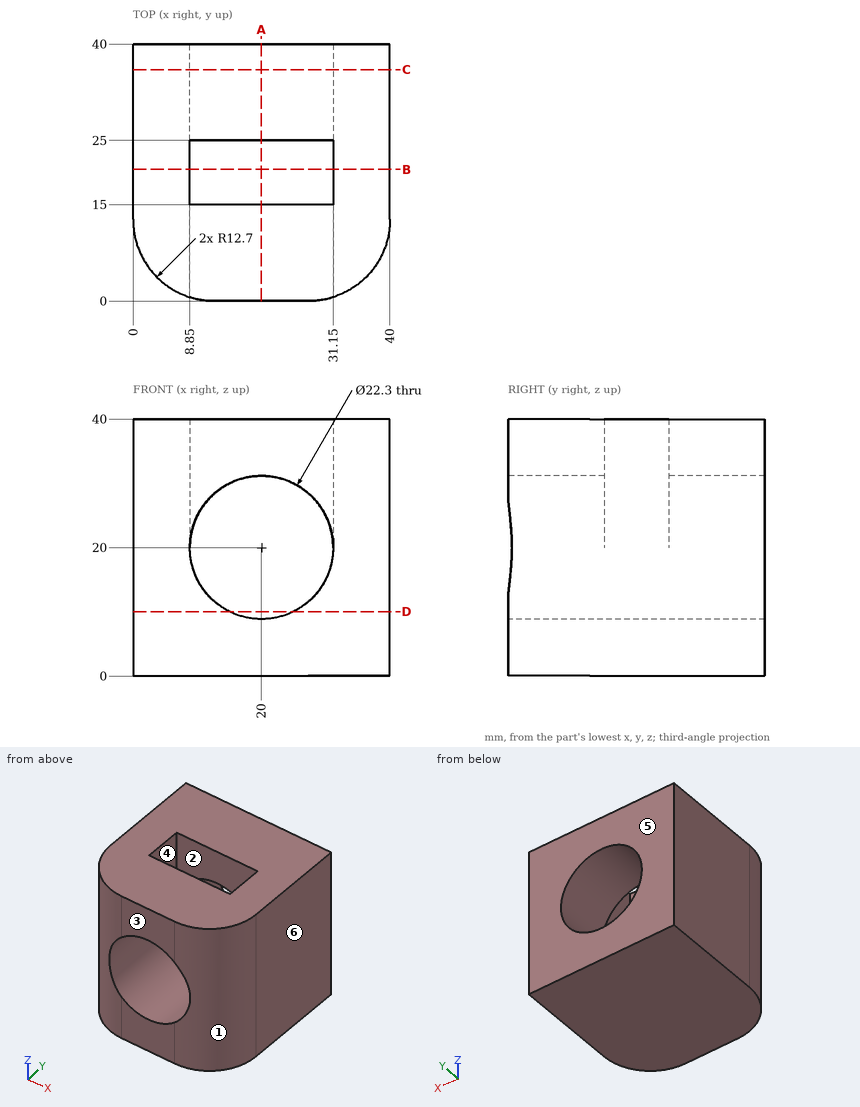
Design review of the part shown in the three views and the two pictorial views. Dimensions are in mm from the part's minimum x, y and z. A direction names the side the tool comes from. Coordinates: 2 decimals unless noted, no trailing zeros. Write each loop counter-clockwise with the first axis right and the second up, starting at its lowest first coordinate (ties: lowest second). Pieces come first, ordered by that corner, then holes.
(1) The part is to be moulded in two halves that separate along Y. For the marked faces 3, 4, 5 and 6, say which applies: +Y half, -Y half, draft (parallel to the pull), parting line (faces both ways), or undercut.
(2) Wall thickness on probe 1 along Y at (x, z) = (17.5, 34); probe 2 along Z at (x, y) = (20, 13): over which ranges is each line inside the solid? List them lowest first.
(3) Add section B-B on y = 20.5. Give the boundary of the cut face in (x, z).
(4) Add section C-C on y = 36. Give the boundary of the cut face in (x, z), then the cut area to 3 significant figures.
(5) Add section A-A on x = 20. Give the boundary of the cut face in (y, z).
(6) Add section D-D on z = 10. Give the boundary of the cut face in (x, y).
(7) Tool access review of the marked faces 1 and 2: name each direction out of +Z, -Z, +X, -X, +Y, -Y from which nothing blocks a thin tool from reaching the whole face with its end or side.
Answer sheet:
1. face 3: -Y half
1. face 4: undercut
1. face 5: +Y half
1. face 6: draft
2. probe 1: y = 0 to 15, 25 to 40
2. probe 2: z = 0 to 8.85, 31.15 to 40
3. outline: (0, 0) - (40, 0) - (40, 40) - (31.15, 40) - (31.15, 20) arc R11.15 cw to (8.85, 20) - (8.85, 40) - (0, 40) - close
4. outline: (0, 0) - (40, 0) - (40, 40) - (0, 40) - close; hole circle Ø22.3 at (20, 20)
4. area: 1,210 mm2
5. outline: (0, 0) - (40, 0) - (40, 8.85) - (0, 8.85) - close; (0, 31.15) - (15, 31.15) - (15, 40) - (0, 40) - close; (25, 31.15) - (40, 31.15) - (40, 40) - (25, 40) - close
6. outline: (0, 12.7) arc R12.7 ccw to (12.7, 0) - (15.07, 0) - (15.07, 40) - (0, 40) - close; (24.93, 0) - (27.3, 0) arc R12.7 ccw to (40, 12.7) - (40, 40) - (24.93, 40) - close
7. face 1: +Z, -Z, +X, -Y
7. face 2: +Z
